Job drawing, mm, ordinate dimensions from the low corner. One solid piece. Round coordinates to 2 decimals unless told otherwise and drop trailing zeros. Loops run counter-clockwise (first coordinate to the right, second up) from the corner with the lowest first, then second, coordinate; pieces in that order, holes last. Notation, with made-up numbers: M 19,33.25 L 62,33.25 A23 cw 62,70.25 Z; hole C 75.25,-31.5 d9. An arc over 180 degrees is marked long. Use a Markdown table: item, result. Add a question column.
(1) Band-saw the part on B-B, the plane y = 0.8. Write the cut outline in (x, z), and give its area (3 significant figures).
(2) Band-saw the part on A-A, the plane x = 16. Write the cut outline in (y, z), and give its area (3 significant figures).
(3) Wall check: L1, parallel to X at y = 0.2, z = 8; L2, parallel to X at y = 0.3, z = 72; L3, parallel to X at y = 1.1, z = 34. Give the ranges that are in metal, low to high.
(4) Band-saw the part on D-D, the plane z = 8. Write the cut outline in (x, y), and give its area (3 significant figures).
(5) Band-saw the part on C-C, the plane z = 72. Write the cut outline in (x, y), and give its area (3 significant figures).
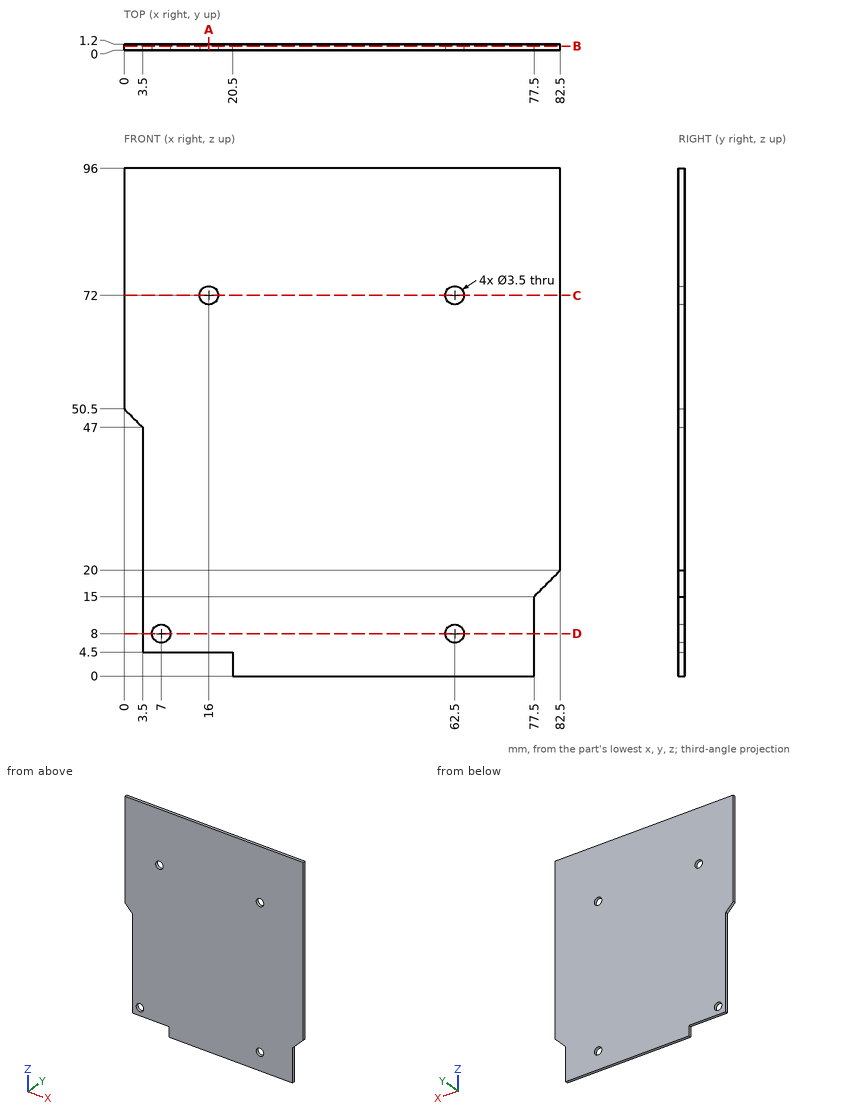
Return value:
| question | item | result |
|---|---|---|
| 1 | outline | M 0,50.5 L 3.5,47 L 3.5,4.5 L 20.5,4.5 L 20.5,0 L 77.5,0 L 77.5,15 L 82.5,20 L 82.5,96 L 0,96 Z; hole C 7,8 d3.5; hole C 16,72 d3.5; hole C 62.5,8 d3.5; hole C 62.5,72 d3.5 |
| 1 | area | 7,550 mm^2 |
| 2 | outline | M 0,4.5 L 1.2,4.5 L 1.2,70.25 L 0,70.25 Z; M 0,73.75 L 1.2,73.75 L 1.2,96 L 0,96 Z |
| 2 | area | 106 mm^2 |
| 3 | L1 | 3.5 to 5.25, 8.75 to 60.75, 64.25 to 77.5 |
| 3 | L2 | 0 to 14.25, 17.75 to 60.75, 64.25 to 82.5 |
| 3 | L3 | 3.5 to 82.5 |
| 4 | outline | M 3.5,0 L 5.25,0 L 5.25,1.2 L 3.5,1.2 Z; M 8.75,0 L 60.75,0 L 60.75,1.2 L 8.75,1.2 Z; M 64.25,0 L 77.5,0 L 77.5,1.2 L 64.25,1.2 Z |
| 4 | area | 80.4 mm^2 |
| 5 | outline | M 0,0 L 14.25,0 L 14.25,1.2 L 0,1.2 Z; M 17.75,0 L 60.75,0 L 60.75,1.2 L 17.75,1.2 Z; M 64.25,0 L 82.5,0 L 82.5,1.2 L 64.25,1.2 Z |
| 5 | area | 90.6 mm^2 |
